from build123d import *


with BuildPart() as part:
    # 草图1 → 旋转1 (revolve)
    with BuildSketch(Plane.XY, mode=Mode.PRIVATE) as revolve_1_sk:
        Polygon((19, 0), (21, 0), (21, 2.5), (20.5, 2.5), (20.5, 3.5), (25.4, 3.5), (25.4, 12.5), (20.5, 12.5), (20.5, 7), (21.1, 7), (21.1, 6), (20, 6), (20, 4.5), (19, 4.5), align=None)
    revolve(revolve_1_sk.sketch.rotate(Axis((0, 0, 0), (0, 1, 0)), 90), axis=Axis((0, 0, 0), (0, 1, 0)))  # turned: the seam where the file's is


solid = part.part
Here's how the part is built. I have some questions about the finished solid (model axes, mm). A direction names the side the tool comes from. Coordinates: 2 decimals unless noted, no trailing zeros. Write each loop counter-clockwise with the first axis right and the second up, starting at its lowest first coordinate (ties: lowest second). Pieces come first, ordered by that corner, then holes.
Item 1: I want a section at A-A on x = 0. Write out the boundary of the cut face in (y, z).
Item 2: On a 3-axis mill with a long thin cutter (end or side, diameter ignored), from which of +Z, -Z, +X, -X, +Y, -Y can I reach the whole of each face in a straight line? I mean faces 1 (the cylindrical face through (7.852, 3.007, -18.937)), 2 (the cylindrical face through (18.548, 2.218, 4.119)), 3 (the cylindrical face through (-6.31, 1.27, -20.03)), 4 (the flat face through (11, 0, -16)), 5 (the cylindrical face through (-0.88, 5.24, 19.98)). Say none if no direction works.
Item 3: Will these pins go through, and if not, where does the flat tip stop? pin 1 (4 mm diameter, centred on y = 10, z = -15.5, fed in from -X); pin 2 (8 mm diameter, centred on x = 20, z = -16, fed in from -Y); pin 3 (20 mm diameter, centred on x = -5, z = 3.5, fed in from +Y); pin 4 (1.5 mm diameter, centred on y = 6.5, z = -20, fed in from +X).
Item 4: If I drill on line 1 (X direction, y = 1.2, z = 0); line 2 (X direction, y = 9.2, z = 0); line 3 (Y direction, x = -1, z = 21.5), over which ranges is the centre line in solid material (lowest first)?
Item 5: If we mould it in two halves opening along Y, with no side actions, what happens to faces 6 (the cylindrical face through (7.852, 9.712, -18.937)), 7 (the flat face through (-21, 12.5, -2)), 8 (the cylindrical face through (-6.338, 6.493, -20.126))? For each: +Y half, -Y half, draft (parallel to the pull), parting line (faces both ways), or undercut.
Item 6: I want a section at B-B on z = 0. Write out the boundary of the cut face in (x, y).
Findings below:
1. outline: (0, -21) - (2.5, -21) - (2.5, -20.5) - (3.5, -20.5) - (3.5, -25.4) - (12.5, -25.4) - (12.5, -20.5) - (7, -20.5) - (7, -21.1) - (6, -21.1) - (6, -20) - (4.5, -20) - (4.5, -19) - (0, -19) - close; (0, 19) - (4.5, 19) - (4.5, 20) - (6, 20) - (6, 21.1) - (7, 21.1) - (7, 20.5) - (12.5, 20.5) - (12.5, 25.4) - (3.5, 25.4) - (3.5, 20.5) - (2.5, 20.5) - (2.5, 21) - (0, 21) - close
2. face 1: none
2. face 2: +Y, -Y
2. face 3: -Y
2. face 4: +Z, -Z, +X, -X, -Y
2. face 5: +Y
3. pin 1: stops at x = -21.52
3. pin 2: stops at y = 3.5
3. pin 3: passes through
3. pin 4: stops at x = 16.57
4. line 1: x = -21 to -19, 19 to 21
4. line 2: x = -25.4 to -20.5, 20.5 to 25.4
4. line 3: y = 3.5 to 12.5
5. face 6: draft
5. face 7: +Y half
5. face 8: undercut
6. outline: (-25.4, 3.5) - (-20.5, 3.5) - (-20.5, 2.5) - (-21, 2.5) - (-21, 0) - (-19, 0) - (-19, 4.5) - (-20, 4.5) - (-20, 6) - (-21.1, 6) - (-21.1, 7) - (-20.5, 7) - (-20.5, 12.5) - (-25.4, 12.5) - close; (19, 0) - (21, 0) - (21, 2.5) - (20.5, 2.5) - (20.5, 3.5) - (25.4, 3.5) - (25.4, 12.5) - (20.5, 12.5) - (20.5, 7) - (21.1, 7) - (21.1, 6) - (20, 6) - (20, 4.5) - (19, 4.5) - close
